For this review, use the dimensioned drawing (mm, ordinates from the lowest corner) and the shaded views. A direction names the side the tool comes from. Round coordinates to 2 decimals unless told otherwise and drop trailing zeros. Loops run counter-clockwise (first coordinate to the right, second up) from the corner with the lowest first, then second, coordinate; pieces in that order, holes last.
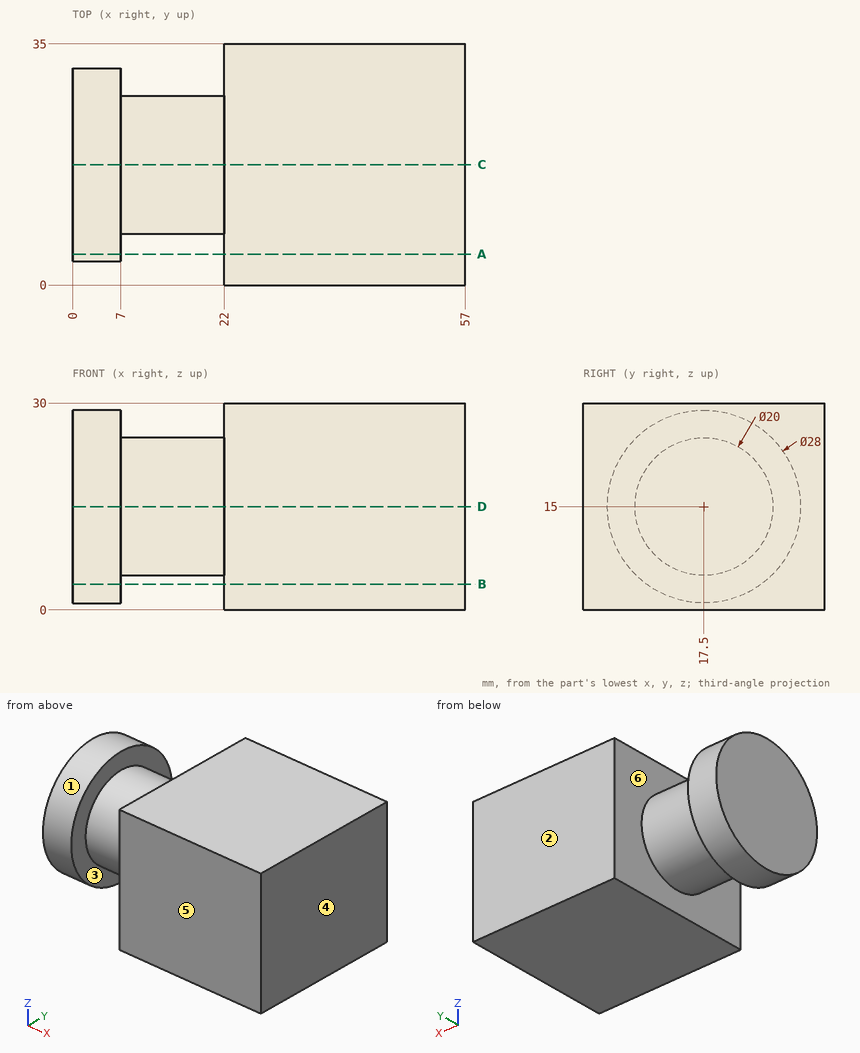
(1) For the marked faces 1, 2 and 3, list the 3-axis set-ups (+Z, -Z, +X, -X, +Y, -Y) from which the entire face can be reached by the end or side of a thin tool; tool diameter is ignored.
(2) Insertion check: pin 1 Ø2 at (x, y) = (19.5, 14) entering from -Z. The pin has a flat end and moves straight along its axis. Give the tip position at first contact, or say it passes through.
(3) For L1, parallel to Z at x = 2, y = 17; L2, parallel to Y at x = 3.5, z = 8.75; L3, parallel to Z at x = 18, y = 22.5, list the stretches that pass through material, from the lowest coordinate up.
(4) Add section D-D (z = 15). Give the boundary of the cut face in (x, y), plus the area to 3 significant figures.
(5) Add section C-C (y = 17.5). Give the boundary of the cut face in (x, z), plus the area to 3 significant figures.
(6) Add section A-A (y = 4.5). Give the boundary of the cut face in (x, z).
(7) The part is to be moulded in two halves that separate along X. For the marked faces 4, 5 and 6, say which applies: pulls with the +X half, pulls with the -X half, needs draft (parallel to the pull), parting line crosses it, or undercut.
(8) Add section B-B (z = 3.75). Give the boundary of the cut face in (x, y), plus the area to 3 significant figures.
Outcome:
1. face 1: -X
1. face 2: +Z, -Z, +X, -X, +Y
1. face 3: none
2. pin 1: stops at z = 5.32
3. L1: z = 1.01 to 28.99
3. L2: y = 4.97 to 30.03
3. L3: z = 6.34 to 23.66
4. outline: (0, 3.5) - (7, 3.5) - (7, 7.5) - (22, 7.5) - (22, 0) - (57, 0) - (57, 35) - (22, 35) - (22, 27.5) - (7, 27.5) - (7, 31.5) - (0, 31.5) - close
4. area: 1,720 mm2
5. outline: (0, 1) - (7, 1) - (7, 5) - (22, 5) - (22, 0) - (57, 0) - (57, 30) - (22, 30) - (22, 25) - (7, 25) - (7, 29) - (0, 29) - close
5. area: 1,550 mm2
6. outline: (0, 9.8) - (7, 9.8) - (7, 20.2) - (0, 20.2) - close; (22, 0) - (57, 0) - (57, 30) - (22, 30) - close
7. face 4: pulls with the +X half
7. face 5: needs draft
7. face 6: undercut
8. outline: (0, 9.17) - (7, 9.17) - (7, 25.83) - (0, 25.83) - close; (22, 0) - (57, 0) - (57, 35) - (22, 35) - close
8. area: 1,340 mm2
